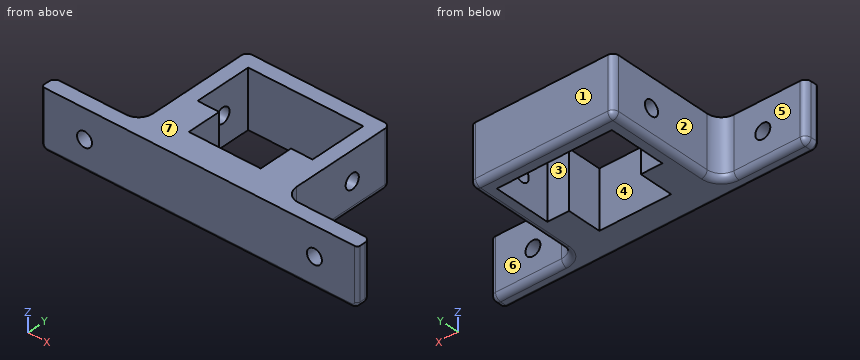
```python
from build123d import *

# Parameters (mm, degrees)
PAD_DEPTH            = 20
SKETCH001_R          = 2.6
POCKET_DEPTH         = 5
SKETCH002_R          = 2.6
POCKET001_DEPTH      = 35.001
POCKET001_DEPTH_BACK = -75.001
FILLET_R             = 5
FILLET001_R          = 2
FILLET002_R          = 2
FILLET003_R          = 1


with BuildPart() as part:
    # Sketch → Pad (new body)
    with BuildSketch(Plane.XY):
        Polygon((-55, 0), (-55, 5), (-25, 5), (-25, 47), (25, 47), (25, 5), (55, 5), (55, 0), align=None)
        Polygon((-20, 42), (-20, 22), (-12.5, 22), (-12.5, 10), (12.5, 10), (12.5, 22), (20, 22), (20, 42), align=None, mode=Mode.SUBTRACT)
    extrude(amount=PAD_DEPTH)

    # Sketch001 (on Face6 of Pad) → Pocket (cut)
    with BuildSketch(Plane(origin=(0, 5, 0), x_dir=(-1, 0, 0), z_dir=(0, 1, 0))):
        with Locations((-40, 10)):
            Circle(SKETCH001_R)
        with Locations((40, 10)):
            Circle(SKETCH001_R)
    extrude(amount=-POCKET_DEPTH, mode=Mode.SUBTRACT)

    # Sketch002 (on Face19 of Pocket) → Pocket001 (cut, two sides)
    with BuildSketch(Plane(origin=(20, 0, 0), x_dir=(0, -1, 0), z_dir=(-1, 0, 0))) as pocket001_sk:
        with Locations((-32, 10)):
            Circle(SKETCH002_R)
    extrude(amount=-POCKET001_DEPTH, mode=Mode.SUBTRACT)
    extrude(pocket001_sk.sketch, amount=-POCKET001_DEPTH_BACK, mode=Mode.SUBTRACT)

    # Fillet
    fillet_edges = [part.edges().sort_by_distance(p)[0] for p in [
        (25, 5, 10),
        (-25, 5, 10),
    ]]
    fillet(fillet_edges, radius=FILLET_R)

    # Fillet001
    fillet001_edges = [part.edges().sort_by_distance(p)[0] for p in [
        (-55, 5, 10),
        (-25, 47, 10),
        (25, 47, 10),
        (55, 5, 10),
    ]]
    fillet(fillet001_edges, radius=FILLET001_R)

    # Fillet002
    fillet002_edges = [part.edges().sort_by_distance(p)[0] for p in [
        (25, 27.5, 0),
    ]]
    fillet(fillet002_edges, radius=FILLET002_R)

    # Fillet003
    fillet003_edges = [part.edges().sort_by_distance(p)[0] for p in [
        (0, 0, 0),
    ]]
    fillet(fillet003_edges, radius=FILLET003_R)


solid = part.part
```
For this review, take the finished solid that the model builds, in its own axes (mm). Face numbers are marked on the shaded views. A direction names the side the tool comes from. Round coordinates to 2 decimals unless told otherwise and drop trailing zeros. Write each loop counter-clockwise with the first axis right and the second up, starting at its lowest first coordinate (ties: lowest second). Pieces come first, ordered by that corner, then holes. Notation, with made-up numbers: (49.25, -6.5) - (97.25, -6.5) arc R14 cw to (97.25, 3.5) - close; hole circle Ø3 at (50, 32.25). An arc over 180 degrees is marked (long way). Answer as a JSON object with one key per item and string values.
1. We need section C-C on z = 18. Give the boundary of the cut face in (x, y).
Response values:
{"outline": "(-55, 1) arc R1 ccw to (-54, 0) - (54, 0) arc R1 ccw to (55, 1) - (55, 3) arc R2 ccw to (53, 5) - (30, 5) arc R5 cw to (25, 10) - (25, 45) arc R2 ccw to (23, 47) - (-23, 47) arc R2 ccw to (-25, 45) - (-25, 10) arc R5 cw to (-30, 5) - (-53, 5) arc R2 ccw to (-55, 3) - close; hole (-20, 22) - (-12.5, 22) - (-12.5, 10) - (12.5, 10) - (12.5, 22) - (20, 22) - (20, 42) - (-20, 42) - close"}
2. Tool access review of the marked faces 4, 5, 6 and 7: name each direction out of +Z, -Z, +X, -X, +Y, -Y from which nothing blocks a thin tool from reaching the whole face with its end or side.
Response values:
{"face 4": "+Z, -Z", "face 5": "+Z, -Z, -X, +Y", "face 6": "+Z, -Z, +X, +Y", "face 7": "+Z, +X, -X, +Y, -Y"}
3. Draft analysis for pull direction X (two halves, no side actions). For the marked faces 1, 2 and 3, state which applies: +X half, -X half, draft (parallel to the pull), parting line (faces both ways), or undercut.
Response values:
{"face 1": "draft", "face 2": "-X half", "face 3": "undercut"}
4. For pin 1 Ø7 at (y, z) = (32, 10) entering from +X; pin 2 Ø5 at (x, z) = (34.5, 15.5) entering from +Y; pin 3 Ø6 at (x, z) = (27.5, 17) entering from +Y; pin 4 Ø3 at (x, z) = (40, 10) entering from -Y, all flat-tipped, find the tip position at first contact; note any pin that passes through.
Response values:
{"pin 1": "stops at x = 25", "pin 2": "stops at y = 5", "pin 3": "stops at y = 46.32", "pin 4": "passes through"}
5. To check wall thickness, follow line 1 along X through (y, z) = (26, 4.75); line 2 along X through (y, z) = (20, 18.25); line 3 along Y through (x, z) = (18, 18.75). State the ranges of each line that lie inside material, in increasing order.
Response values:
{"line 1": "x = -25 to -20, 20 to 25", "line 2": "x = -25 to -12.5, 12.5 to 25", "line 3": "y = 0 to 22, 42 to 47"}
6. We need section D-D on y = 17. Give the boundary of the cut face in (x, z).
Response values:
{"outline": "(-25, 2) arc R2 ccw to (-23, 0) - (-12.5, 0) - (-12.5, 20) - (-25, 20) - close; (12.5, 0) - (23, 0) arc R2 ccw to (25, 2) - (25, 20) - (12.5, 20) - close"}
7. We need section A-A on y = 32. Give the boundary of the cut face in (x, z).
Response values:
{"outline": "(-25, 2) arc R2 ccw to (-23, 0) - (-20, 0) - (-20, 7.4) - (-25, 7.4) - close; (-25, 12.6) - (-20, 12.6) - (-20, 20) - (-25, 20) - close; (20, 0) - (23, 0) arc R2 ccw to (25, 2) - (25, 7.4) - (20, 7.4) - close; (20, 12.6) - (25, 12.6) - (25, 20) - (20, 20) - close"}
8. We need section B-B on x = -40. Give the boundary of the cut face in (y, z).
Response values:
{"outline": "(0, 1) arc R1 ccw to (1, 0) - (3, 0) arc R2 ccw to (5, 2) - (5, 7.4) - (0, 7.4) - close; (0, 12.6) - (5, 12.6) - (5, 20) - (0, 20) - close"}
